```python
from build123d import *

# Parameters (mm, degrees)
SKETCH_1_W           = 60
SKETCH_1_H           = 60
EXTRUDE_1_DEPTH      = 7
SKETCH_2_W           = 18
SKETCH_2_H           = 60
SKETCH_2_R           = 3
EXTRUDE_2_DEPTH      = 15
SKETCH_3_W           = 43
SKETCH_3_H           = 70
CUT_EXTRUDE_1_DEPTH  = 7
SKETCH_4_W           = 24
SKETCH_4_H           = 60
EXTRUDE_3_DEPTH      = 15
SKETCH_12_W          = 24
SKETCH_12_H          = 12
CUT_EXTRUDE_8_DEPTH  = 87
FILLET_START         = -16
FILLET_8_DEPTH       = 24
CHAMFER_23_SIZE      = 1
CHAMFER_24_SIZE      = 1
EXTRUDE_4_DEPTH      = 7
EXTRUDE_5_DEPTH      = 7
SKETCH_23_W          = 24
SKETCH_23_H          = 60
CUT_EXTRUDE_9_DEPTH  = 11
SKETCH_24_R          = 11.5
SKETCH_24_R_2        = 1.6
CUT_EXTRUDE_10_DEPTH = 34
SKETCH_25_R          = 3
CUT_EXTRUDE_11_DEPTH = 3
CHAMFER_25_SIZE      = 2
CHAMFER_26_SIZE      = 1
CHAMFER_27_SIZE      = 1
CHAMFER_28_SIZE      = 1
SKETCH_26_W          = 14
SKETCH_26_H          = 14
CUT_EXTRUDE_12_DEPTH = 12
SKETCH_28_R          = 3.1
CUT_EXTRUDE_13_DEPTH = 15
SKETCH_30_R          = 3
CUT_EXTRUDE_14_DEPTH = 10
SKETCH_31_R          = 3.1
CUT_EXTRUDE_15_DEPTH = 35


with BuildPart() as part:
    # 草图1 → 凸台-拉伸1 (new body)
    with BuildSketch(Plane(origin=(0, 0, 0), x_dir=(1, 0, 0), z_dir=(0, 1, 0))):
        Rectangle(SKETCH_1_W, SKETCH_1_H)
    extrude(amount=EXTRUDE_1_DEPTH)

    # 草图2 → 凸台-拉伸2 (add)
    # profile 1 of 2: a face of its own
    with BuildSketch(Plane.XZ):
        with Locations((-21, 0)):
            Rectangle(SKETCH_2_W, SKETCH_2_H)
        with Locations(Location((-21, 21, 0), (0, 0, 270))):
            Circle(SKETCH_2_R, mode=Mode.SUBTRACT)
        with Locations(Location((-21, -21, 0), (0, 0, 270))):
            Circle(SKETCH_2_R, mode=Mode.SUBTRACT)
    # profile 2 of 2: a face of its own
    with BuildSketch(Plane.XZ):
        with Locations((21, 0)):
            Rectangle(SKETCH_2_W, SKETCH_2_H)
        with Locations(Location((21, -21, 0), (0, 0, 90))):
            Circle(SKETCH_2_R, mode=Mode.SUBTRACT)
        with Locations(Location((21, 21, 0), (0, 0, 90))):
            Circle(SKETCH_2_R, mode=Mode.SUBTRACT)
    extrude(amount=EXTRUDE_2_DEPTH)

    # 草图3 → 切除-拉伸1 (cut)
    with BuildSketch(Plane(origin=(0, 7, 0), x_dir=(1, 0, 0), z_dir=(0, 1, 0))):
        with Locations((0, 30)):
            Rectangle(SKETCH_3_W, SKETCH_3_H)
    extrude(amount=-CUT_EXTRUDE_1_DEPTH, mode=Mode.SUBTRACT)

    # 草图4 → 凸台-拉伸3 (add)
    with BuildSketch(Plane.XZ):
        Rectangle(SKETCH_4_W, SKETCH_4_H)
    extrude(amount=EXTRUDE_3_DEPTH)

    # 草图12 → 切除-拉伸8 (cut)
    with BuildSketch(Plane(origin=(0, 0, -30), x_dir=(-1, 0, 0), z_dir=(0, 0, -1))):
        with Locations((0, -15)):
            Rectangle(SKETCH_12_W, SKETCH_12_H)
    extrude(amount=-CUT_EXTRUDE_8_DEPTH, mode=Mode.SUBTRACT)

    # 圆角8: read off the stored shape, not the designer's step
    # 圆角8 outline → 圆角8 (cut)
    with BuildSketch(Plane(origin=(0, 0, 0), x_dir=(1, 0, 0), z_dir=(0, 1, 0)).offset(FILLET_START)):
        with BuildLine():
            Line((-30, 30), (-30, 21))
            ThreePointArc((-30, 21), (-27.363961031, 27.363961031), (-21, 30))
            Line((-21, 30), (-30, 30))
        make_face()
        with BuildLine():
            ThreePointArc((-21, -30), (-27.363961031, -27.363961031), (-30, -21))
            Line((-30, -21), (-30, -30))
            Line((-30, -30), (-21, -30))
        make_face()
        with BuildLine():
            Line((30, 30), (21, 30))
            ThreePointArc((21, 30), (27.363961031, 27.363961031), (30, 21))
            Line((30, 21), (30, 30))
        make_face()
        with BuildLine():
            ThreePointArc((30, -21), (27.363961031, -27.363961031), (21, -30))
            Line((21, -30), (30, -30))
            Line((30, -30), (30, -21))
        make_face()
    extrude(amount=FILLET_8_DEPTH, mode=Mode.SUBTRACT)

    # 倒角23
    chamfer_23_edges = [part.edges().sort_by_distance(p)[0] for p in [
        (-21, -15, 24),
        (-21, -15, -18),
        (21, -15, -24),
        (21, -15, 18),
    ]]
    chamfer(chamfer_23_edges, length=CHAMFER_23_SIZE)

    # 倒角24
    chamfer_24_edges = [part.edges().sort_by_distance(p)[0] for p in [
        (-30, -15, 0),
        (-16.5, -15, -30),
        (-27.363961031, -15, 27.363961031),
        (-27.363961031, -15, -27.363961031),
        (30, -15, 0),
        (16.5, -15, 30),
        (27.363961031, -15, 27.363961031),
        (27.363961031, -15, -27.363961031),
        (16.5, -15, -30),
        (-16.5, -15, 30),
    ]]
    chamfer(chamfer_24_edges, length=CHAMFER_24_SIZE)

    # 草图21 → 凸台-拉伸4 (add)
    with BuildSketch(Plane(origin=(0, 0, 0), x_dir=(1, 0, 0), z_dir=(0, 1, 0))):
        with BuildLine():
            Line((-21.5, 23.958039892), (-21.5, 18.041960108))
            Line((-21.5, 18.041960108), (-21.5, -5))
            Line((-21.5, -5), (21.5, -5))
            Line((21.5, -5), (21.5, 18.041960108))
            Line((21.5, 18.041960108), (21.5, 23.958039892))
            Line((21.5, 23.958039892), (21.5, 29.986100378))
            ThreePointArc((21.5, 29.986100378), (21.250096581, 29.996524423), (21, 30))
            Line((21, 30), (-21, 30))
            ThreePointArc((-21, 30), (-21.250096581, 29.996524423), (-21.5, 29.986100378))
            Line((-21.5, 29.986100378), (-21.5, 23.958039892))
        make_face()
    extrude(amount=EXTRUDE_4_DEPTH)

    # 草图22 → 凸台-拉伸5 (add)
    with BuildSketch(Plane(origin=(0, 7, 0), x_dir=(1, 0, 0), z_dir=(0, 1, 0))):
        with BuildLine():
            Line((21, 30), (-21, 30))
            ThreePointArc((-21, 30), (-27.363961031, 27.363961031), (-30, 21))
            Line((-30, 21), (-30, -21))
            ThreePointArc((-30, -21), (-27.363961031, -27.363961031), (-21, -30))
            Line((-21, -30), (21, -30))
            ThreePointArc((21, -30), (27.363961031, -27.363961031), (30, -21))
            Line((30, -21), (30, 21))
            ThreePointArc((30, 21), (27.363961031, 27.363961031), (21, 30))
        make_face()
    extrude(amount=EXTRUDE_5_DEPTH)

    # 草图23 → 切除-拉伸9 (cut)
    with BuildSketch(Plane.XZ.offset(9)):
        Rectangle(SKETCH_23_W, SKETCH_23_H)
    extrude(amount=-CUT_EXTRUDE_9_DEPTH, mode=Mode.SUBTRACT)

    # 草图24 → 切除-拉伸10 (cut)
    with BuildSketch(Plane(origin=(0, 14, 0), x_dir=(1, 0, 0), z_dir=(0, 1, 0))):
        with Locations(Location((0, 0, 0), (0, 0, 270))):
            Circle(SKETCH_24_R)
        with Locations(Location((15.5, 15.5, 0), (0, 0, 270))):
            Circle(SKETCH_24_R_2)
        with Locations(Location((15.429289322, -15.429289322, 0), (0, 0, 270))):
            Circle(SKETCH_24_R_2)
        with Locations(Location((-15.5, -15.358578644, 0), (0, 0, 270))):
            Circle(SKETCH_24_R_2)
        with Locations(Location((-15.429289322, 15.570710678, 0), (0, 0, 270))):
            Circle(SKETCH_24_R_2)
    extrude(amount=-CUT_EXTRUDE_10_DEPTH, mode=Mode.SUBTRACT)

    # 草图25 → 切除-拉伸11 (cut)
    with BuildSketch(Plane.XZ.offset(15)):
        with Locations(Location((15.5, -15.5, 0), (0, 0, 270))):
            Circle(SKETCH_25_R)
        with Locations(Location((-15.5, -15.5, 0), (0, 0, 270))):
            Circle(SKETCH_25_R)
        with Locations(Location((-15.5, 15.5, 0), (0, 0, 270))):
            Circle(SKETCH_25_R)
        with Locations(Location((15.5, 15.5, 0), (0, 0, 270))):
            Circle(SKETCH_25_R)
    extrude(amount=-CUT_EXTRUDE_11_DEPTH, mode=Mode.SUBTRACT)

    # 倒角25
    chamfer_25_edges = [part.edges().sort_by_distance(p)[0] for p in [
        (27.363961031, 14, -27.363961031),
        (0, 14, -30),
        (-27.363961031, 14, -27.363961031),
        (-30, 14, 0),
        (-27.363961031, 14, 27.363961031),
        (0, 14, 30),
        (27.363961031, 14, 27.363961031),
        (30, 14, 0),
    ]]
    chamfer(chamfer_25_edges, length=CHAMFER_25_SIZE)

    # 倒角26
    # the kernel refuses this chamfer: 1 mm, written as the material it adds along each edge
    with BuildSketch(Plane(origin=(12, 2, -30), x_dir=(0, -1, 0), z_dir=(0, 0, 1))) as chamfer_26_piece_1_section:
        Polygon((CHAMFER_26_SIZE, 0), (0, -CHAMFER_26_SIZE), (0, 0), align=None)
    chamfer_26_piece_1 = extrude(amount=60, mode=Mode.PRIVATE)
    chamfer_26_piece_1 = chamfer_26_piece_1 - Plane(origin=(0, 2, 0), x_dir=(0, 0, 1), z_dir=(0, 1, 0)) * Cylinder(11.5, 124, mode=Mode.PRIVATE)
    add(chamfer_26_piece_1)
    with BuildSketch(Plane(origin=(-12, 2, 30), x_dir=(1, 0, 0), z_dir=(0, 0, -1))) as chamfer_26_piece_2_section:
        Polygon((CHAMFER_26_SIZE, 0), (0, CHAMFER_26_SIZE), (0, 0), align=None)
    chamfer_26_piece_2 = extrude(amount=60, mode=Mode.PRIVATE)
    chamfer_26_piece_2 = chamfer_26_piece_2 - Plane(origin=(0, 2, 0), x_dir=(0, 0, 1), z_dir=(0, 1, 0)) * Cylinder(11.5, 124, mode=Mode.PRIVATE)
    add(chamfer_26_piece_2)
    # the kernel refuses this chamfer: 1 mm, written as the material it takes off along each edge
    with BuildSketch(Plane(origin=(-12, -15, 31.571682988), x_dir=(-1, 0, 0), z_dir=(0, 0, -1)), Plane(origin=(12, -15, -31.571682988), x_dir=(1, 0, 0), z_dir=(0, 0, 1))) as chamfer_26_2_piece_1:
        Polygon((CHAMFER_26_SIZE, 0), (0, CHAMFER_26_SIZE), (0, 0), align=None)
    extrude(amount=63.143365976, mode=Mode.SUBTRACT)

    # 倒角27
    chamfer_27_edges = [part.edges().sort_by_distance(p)[0] for p in [
        (-12, -6.5, -30),
        (0, 2, -30),
        (12, -6.5, -30),
        (11.5, 1.5, -30),
        (-11.5, 1.5, -30),
    ]]
    chamfer(chamfer_27_edges, length=CHAMFER_27_SIZE)

    # 倒角28
    chamfer_28_edges = [part.edges().sort_by_distance(p)[0] for p in [
        (-12, -6.5, 30),
        (0, 2, 30),
        (12, -6.5, 30),
        (11.5, 1.5, 30),
    ]]
    chamfer(chamfer_28_edges, length=CHAMFER_28_SIZE)

    # 草图26 → 切除-拉伸12 (cut)
    with BuildSketch(Plane.XZ.offset(15)):
        with Locations((12, 0)):
            Rectangle(SKETCH_26_W, SKETCH_26_H)
    extrude(amount=-CUT_EXTRUDE_12_DEPTH, mode=Mode.SUBTRACT)

    # 草图28 → 切除-拉伸13 (cut)
    with BuildSketch(Plane.XZ.offset(15)):
        with Locations(Location((-21, 21, 0), (0, 0, 270))):
            Circle(SKETCH_28_R)
        with Locations(Location((21, 21, 0), (0, 0, 270))):
            Circle(SKETCH_28_R)
        with Locations(Location((21, -21, 0), (0, 0, 270))):
            Circle(SKETCH_28_R)
        with Locations(Location((-21, -21, 0), (0, 0, 270))):
            Circle(SKETCH_28_R)
    extrude(amount=-CUT_EXTRUDE_13_DEPTH, mode=Mode.SUBTRACT)

    # 草图30 → 切除-拉伸14 (cut)
    with BuildSketch(Plane.XZ.offset(12)):
        with Locations(Location((-15.5, 15.5, 0), (0, 0, 270))):
            Circle(SKETCH_30_R)
        with Locations(Location((15.5, 15.5, 0), (0, 0, 270))):
            Circle(SKETCH_30_R)
        with Locations(Location((15.5, -15.5, 0), (0, 0, 270))):
            Circle(SKETCH_30_R)
        with Locations(Location((-15.5, -15.5, 0), (0, 0, 270))):
            Circle(SKETCH_30_R)
    extrude(amount=-CUT_EXTRUDE_14_DEPTH, mode=Mode.SUBTRACT)

    # 草图31 → 切除-拉伸15 (cut)
    with BuildSketch(Plane.XZ):
        with Locations(Location((-21, 21, 0), (0, 0, 270))):
            Circle(SKETCH_31_R)
        with Locations(Location((21, 21, 0), (0, 0, 270))):
            Circle(SKETCH_31_R)
        with Locations(Location((21, -21, 0), (0, 0, 270))):
            Circle(SKETCH_31_R)
        with Locations(Location((-21, -21, 0), (0, 0, 270))):
            Circle(SKETCH_31_R)
    extrude(amount=-CUT_EXTRUDE_15_DEPTH, mode=Mode.SUBTRACT)


solid = part.part
```
The model under review builds one solid part; all positions refer to its coordinate system, in mm. A direction names the side the tool comes from. Coordinates: 2 decimals unless noted, no trailing zeros. Write each loop counter-clockwise with the first axis right and the second up, starting at its lowest first coordinate (ties: lowest second). Pieces come first, ordered by that corner, then holes.
1) Clearance check with flat-ended pins moving along their axes: pin 1 Ø2 at (x, z) = (17, -2.5) entering from -Y; pin 2 Ø3 at (x, z) = (-16.5, -16.5) entering from -Y; pin 3 Ø1.5 at (x, z) = (6, 11.5) entering from -Y. State where each tip first meets the part, or that it passes through.
2) To check wall thickness, follow probe 1 along X at (y, z) = (-6, 15.5); probe 2 along X at (y, z) = (-1, 21); probe 3 along Z at (x, y) = (20, -12). State the ranges of each line that lie inside material, in increasing order.
3) We need section B-B on z = 0. State the section outline as (x, y) points, then the cut area to 3 significant figures.
4) We need section A-A on y = -13. Count the separate pieces of the cut face and the enclosed holes in it, then the cut area to 3 significant figures.
5) Machinability: for faces 1 (the face through (-14.35, 6.11, -16.75)), 2 (the face through (-17, -2, -17)), 3 (the face through (-11.85, 1.87, -29.51)), which of the approach directions +Z, -Z, +X, -X, +Y, -Y give a long, thin tool a straight path to every point of the face, cutting with its end or side? Answer none if there is none.
6) The part is to be moulded in two halves that separate along Z. For faces 4 (the face through (-12, -7, 0)), 5 (the face through (0, 13, -29)), 6 (the face through (0, 5, 30)), 7 (the face through (19.114, -0.247, -18.54)), say which applies: pulls with the +Z half, pulls with the -Z half, needs draft (parallel to the pull), parting line crosses it, or undercut.
Answer list:
1. pin 1: stops at y = -3
1. pin 2: stops at y = -2
1. pin 3: stops at y = 2
2. probe 1: x = -30 to -18.5, -12.5 to -12, 12 to 12.5, 18.5 to 30
2. probe 2: x = -30 to -24.1, -17.9 to -12, 12 to 17.9, 24.1 to 30
2. probe 3: z = -30 to -23.93, -18.07 to 18.07, 23.93 to 30
3. outline: (-30, -14) - (-29, -15) - (-13, -15) - (-12, -14) - (-12, 1) - (-11.5, 1.5) - (-11.5, 14) - (-28, 14) - (-30, 12) - close; (11.5, 1.5) - (12, 1) - (12, -3) - (19, -3) - (19, -15) - (29, -15) - (30, -14) - (30, 12) - (28, 14) - (11.5, 14) - close
3. area: 967 mm2
4. separate pieces: 2
4. enclosed holes: 8
4. area: 1,760 mm2
5. face 1: +Y, -Y
5. face 2: -Y
5. face 3: -Z, -Y
6. face 4: needs draft
6. face 5: pulls with the -Z half
6. face 6: pulls with the +Z half
6. face 7: undercut
